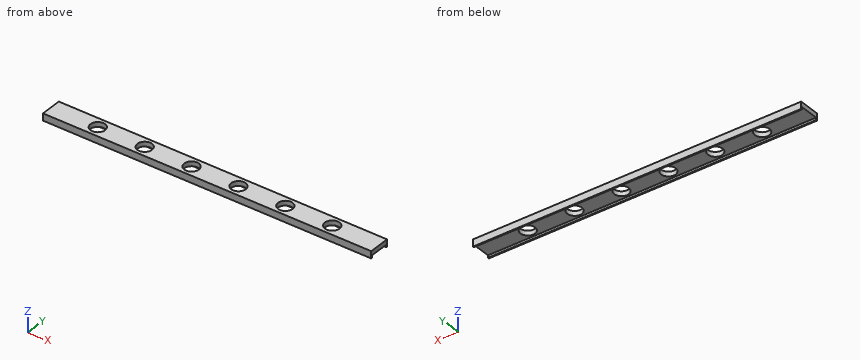
Autodesk Inventor part; units mm, degrees
ref_plane "YZ Plane" through (0, 0, 0) normal (1, 0, 0) x (0, 1, 0)
ref_plane "XZ Plane" through (0, 0, 0) normal (0, 1, 0) x (-1, 0, 0)
ref_plane "XY Plane" through (0, 0, 0) normal (0, 0, 1) x (1, 0, 0)
sketch "Esquisse1" plane through (0, 0, 0) normal (0, 0, 1) x (1, 0, 0)
  line L0 (40, 3.9877) -> (-100, 3.9877)
  line L1 (-100, 3.9877) -> (-100, -4.0123)
  line L2 (-100, -4.0123) -> (40, -4.0123)
  line L3 (40, -4.0123) -> (40, 3.9877)
  circle A0 centre (0, 0) radius 3.125
  line L4 (15.1704, 0) -> (0, 0) construction
  circle A1 centre (-20, 0) radius 3.125
  circle A2 centre (-40, 0) radius 3.125
  circle A3 centre (-60, 0) radius 3.125
  circle A4 centre (-80, 0) radius 3.125
  circle A5 centre (20, 0) radius 3.125
  dimension "d0" = 8
  dimension "d1" = 140
  dimension "d2" = 40
  dimension "d3" = 6.25
  dimension "d6" = 20
  dimension "d13" = 20
extrude "Extrusion1" add sketch "Esquisse1" along normal blind 2
sketch "Esquisse2" plane through (0, 0, 2) normal (0, 0, 1) x (1, 0, 0)
  line L0 (-100, 3.9877) -> (40, 3.9877)
  line L1 (40, 3.9877) -> (40, 4.4877)
  line L2 (40, 4.4877) -> (-100, 4.4877)
  line L3 (-100, 4.4877) -> (-100, 3.9877)
  line L4 (40, -4.0123) -> (-100, -4.0123)
  line L5 (-100, -4.0123) -> (-100, -4.5123)
  line L6 (-100, -4.5123) -> (40, -4.5123)
  line L7 (40, -4.5123) -> (40, -4.0123)
  point P0 (0, 0)
  dimension "d20" = 140
  dimension "d21" = 140
  dimension "d22" = 0.5
  dimension "d23" = 0.5
extrude "Extrusion2" add sketch "Esquisse2" against normal blind 3
properties part number "couvercle"
Geometry: final body of the model. Coordinates: model frame, mm. Give positions to 0.01 mm unless a question says otherwise; leave off trailing zeros. Write each loop counter-clockwise with the first axis right and the second up, starting at its lowest first coordinate (ties: lowest second). Pieces come first, ordered by that corner, then holes. Notation, with made-up numbers: (47, 38) -> (60, 38) arc R20 ccw to (60, 71) -> close; hole circle Ø2 at (30, 67). An arc over 180 degrees is marked (long way). Answer in a Markdown table with one row per item.
(1) Section query C-C on z = -0.45. Return loops of the section in (x, y).
Answers below:
| item | result |
|---|---|
| outline | (-100, -4.51) -> (40, -4.51) -> (40, -4.01) -> (-100, -4.01) -> close; (-100, 3.99) -> (40, 3.99) -> (40, 4.49) -> (-100, 4.49) -> close |
(2) Section query D-D on x = -70.5. Return loops of the section in (y, z), then the cut area to 3 significant figures.
Answers below:
| item | result |
|---|---|
| outline | (-4.51, -1) -> (-4.01, -1) -> (-4.01, 0) -> (3.99, 0) -> (3.99, -1) -> (4.49, -1) -> (4.49, 2) -> (-4.51, 2) -> close |
| area | 19.0 mm^2 |
(3) Section query B-B on y = 0. Return loops of the section in (x, z) (3 decimals).
Answers below:
| item | result |
|---|---|
| outline | (-100, 0) -> (-83.125, 0) -> (-83.125, 2) -> (-100, 2) -> close; (-76.875, 0) -> (-63.125, 0) -> (-63.125, 2) -> (-76.875, 2) -> close; (-56.875, 0) -> (-43.125, 0) -> (-43.125, 2) -> (-56.875, 2) -> close; (-36.875, 0) -> (-23.125, 0) -> (-23.125, 2) -> (-36.875, 2) -> close; (-16.875, 0) -> (-3.125, 0) -> (-3.125, 2) -> (-16.875, 2) -> close; (3.125, 0) -> (16.875, 0) -> (16.875, 2) -> (3.125, 2) -> close; (23.125, 0) -> (40, 0) -> (40, 2) -> (23.125, 2) -> close |
(4) Pin query (flat end, axial travel): pin 1 (1.5 mm diameter, centred on y = 3, z = -0.5, fed in from -X); pin 2 (4 mm diameter, centred on x = -75.5, y = -0.5, fed in from -Z). Return the tip coordinate at first contact, or that it passes through.
Answers below:
| item | result |
|---|---|
| pin 1 | x = -100 |
| pin 2 | z = 0 |
(5) Ray query, line 1 along Y through (x, z) = (0, 0.5) (3 decimals); line 2 along Y through (x, z) = (5, -0.15); line 3 along Z through (x, y) = (-89.5, 3.5). Return the intervals inside material, ascending. Write a range as [from, to].
Answers below:
| item | result |
|---|---|
| line 1 | [-4.512, -3.125], [3.125, 4.488] |
| line 2 | [-4.51, -4.01], [3.99, 4.49] |
| line 3 | [0, 2] |
(6) Section query A-A on x = -40. Return loops of the section in (y, z) (3 decimals), then the cut area to 3 significant figures.
Answers below:
| item | result |
|---|---|
| outline | (-4.512, -1) -> (-4.012, -1) -> (-4.012, 0) -> (-3.125, 0) -> (-3.125, 2) -> (-4.512, 2) -> close; (3.125, 0) -> (3.988, 0) -> (3.988, -1) -> (4.488, -1) -> (4.488, 2) -> (3.125, 2) -> close |
| area | 6.50 mm^2 |
